Could you check a few things on this model? Use its own coordinates, in mm. A direction names the side the tool comes from. Round coordinates to 2 decimals unless told otherwise and drop trailing zeros. Write each loop counter-clockwise with the first axis right and the second up, starting at its lowest first coordinate (ties: lowest second). Pieces come first, ordered by that corner, then holes.
```python
from build123d import *

# Parameters (mm, degrees)
F0_R     = 25.4
F1_DEPTH = 28.575
F2_R     = 22.86
F3_DEPTH = 25.4
F4_W     = 12.7
F4_H     = 12.7
F5_DEPTH = 12.7


with BuildPart() as f1:
    # F0 (on Top) → F1 (new body)
    with BuildSketch(Plane.XY):
        Circle(F0_R)
    extrude(amount=F1_DEPTH)

    # F2 (on face) → F3 (cut)
    with BuildSketch(Plane.XY.offset(28.575)):
        Circle(F2_R)
    extrude(amount=-F3_DEPTH, mode=Mode.SUBTRACT)

    # F4 (on face) → F5 (join)
    with BuildSketch(Plane(origin=(0, 0, 0), x_dir=(1, 0, 0), z_dir=(0, 0, -1))):
        Rectangle(F4_W, F4_H)
    extrude(amount=F5_DEPTH)


solid = f1.part
```
Q1. I'm going to push flat-ended pins straight in: pin 1 Ø6 at (x, z) = (9, 3) entering from +Y; pin 2 Ø14 at (x, z) = (2.5, -5.5) entering from -Y; pin 3 Ø6 at (x, z) = (-15.5, 7.5) entering from +Y. Where does each tip first touch, or does it pass through?
Q2. Imagine slicing it at D-D, the plane y = -10. Write out the boundary of the cut face in (x, z) (3 decimals).
Q3. Imagine slicing it at C-C, the plane z = 2.5. Write out the boundary of the cut face in (x, y), then the cut area to 3 significant figures.
Q4. If I drill on L1, parallel to Y at x = 0, z = 22.25; L2, parallel to Z at x = -3.5, y = 11.5 (3 decimals); L3, parallel to Z at x = 23.5, y = 3 (3 decimals), over which ranges is the centre line in solid material (lowest first)?
Q5. On a 3-axis mill with a long thin cutter (end or side, diameter ignored), from which of +Z, -Z, +X, -X, +Y, -Y can I reach the whole of each face in a straight line? I mean faces 1 (the flat face through (0, 6.35, -6)), 2 (the flat face through (0, 0, 3.175)), 3 (the flat face through (0, -6.35, -6)). Say none if no direction works.
Q6. We'd pull the mould along Y, two halves only. Please class faces 4 (the flat face through (6.35, 0, -6)), 5 (the cylindrical face through (21.804, 6.867, 16.053)), 6 (the cylindrical face through (-5.506, -24.796, 14.087)): pulls with the +Y half, pulls with the -Y half, needs draft (parallel to the pull), parting line crosses it, or undercut.
Q7. Imagine slicing it at A-A, the plane x = 0. Write out the boundary of the cut face in (y, z) (3 decimals).
Results found:
1. pin 1: stops at y = 24.68
1. pin 2: stops at y = -25.4
1. pin 3: stops at y = 22.11
2. outline: (-23.349, 0) - (23.349, 0) - (23.349, 28.575) - (20.557, 28.575) - (20.557, 3.175) - (-20.557, 3.175) - (-20.557, 28.575) - (-23.349, 28.575) - close
3. outline: circle Ø50.8 at (0, 0)
3. area: 2,030 mm2
4. L1: y = -25.4 to -22.86, 22.86 to 25.4
4. L2: z = 0 to 3.175
4. L3: z = 0 to 28.575
5. face 1: -Z, +X, -X, +Y
5. face 2: +Z
5. face 3: -Z, +X, -X, -Y
6. face 4: needs draft
6. face 5: undercut
6. face 6: parting line crosses it
7. outline: (-25.4, 0) - (-6.35, 0) - (-6.35, -12.7) - (6.35, -12.7) - (6.35, 0) - (25.4, 0) - (25.4, 28.575) - (22.86, 28.575) - (22.86, 3.175) - (-22.86, 3.175) - (-22.86, 28.575) - (-25.4, 28.575) - close
